Answer from the drawing. Dimensions are ordinates in mm from the lowest x, y and z of the part. A direction names the side the tool comes from. Coordinates: 2 decimals unless noted, no trailing zeros. Order: outer loops, then holes, each group sorted by start corner. A loop starts at its lowest first (then second) coordinate and runs counter-clockwise, first axis right, second up. Notation, with made-up numbers: M 81,-38 L 92,-38 A15 ccw 92,-22 Z; hole C -14.5,38.5 d1. An arc over 180 degrees is marked long. Write each question's results on one line, items separated by ' | '.
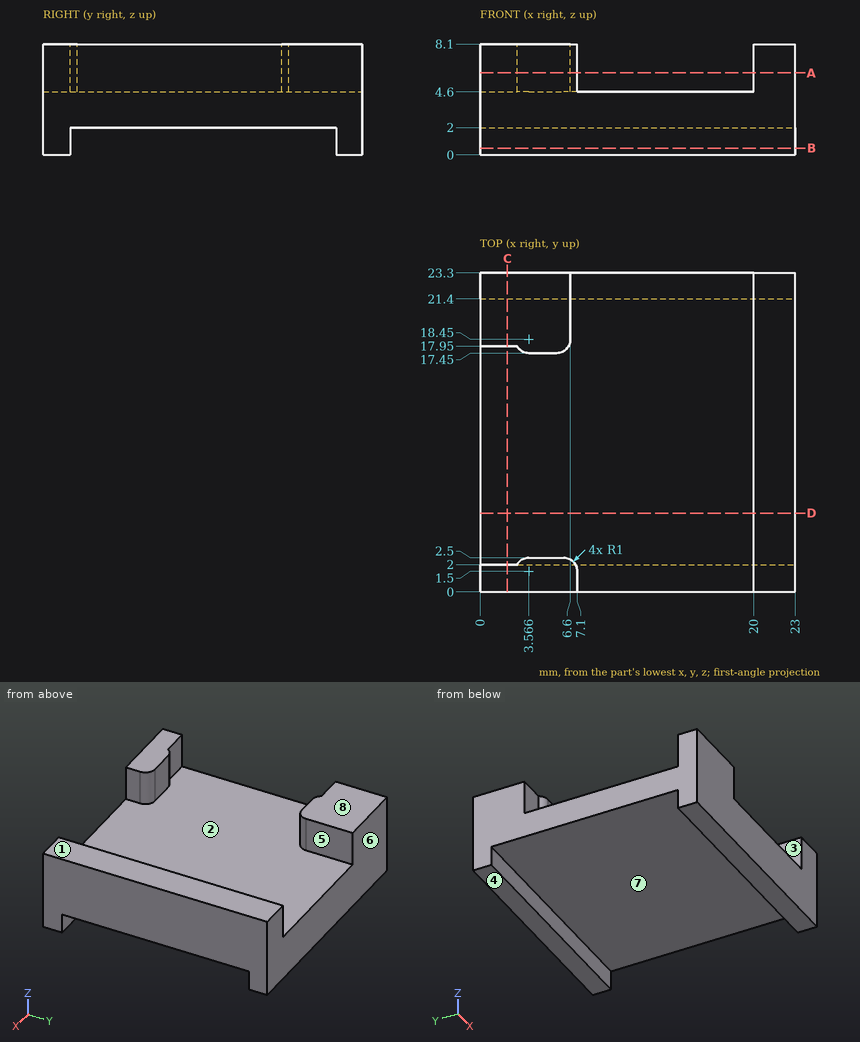
(1) The part is cut by section D-D, the plane y = 5.75. Write down the section's boundary in (x, z).
Conclusion:
outline: M 0,2 L 23,2 L 23,8.1 L 20,8.1 L 20,4.6 L 0,4.6 Z
(2) The part is cut by section A-A, the plane z = 6. Write down the section's boundary in (x, y), then the cut area to 3 significant figures.
Conclusion:
outline: M 0,0 L 7.1,0 L 7.1,1.5 A1 ccw 6.1,2.5 L 3.57,2.5 A1 ccw 2.7,2 L 0,2 Z; M 0,17.95 L 2.7,17.95 A1 ccw 3.57,17.45 L 5.6,17.45 A1 ccw 6.6,18.45 L 6.6,23.3 L 0,23.3 Z; M 20,0 L 23,0 L 23,23.3 L 20,23.3 Z | area: 123 mm²
(3) The part is cut by section B-B, the plane z = 0.5. Write down the section's boundary in (x, y), then the cut area to 3 significant figures.
Conclusion:
outline: M 0,0 L 23,0 L 23,2 L 0,2 Z; M 0,21.4 L 23,21.4 L 23,23.3 L 0,23.3 Z | area: 89.7 mm²
(4) Straight lines are drawn through the part: line 1 (Y direction, x = 3.5, z = 6); line 2 (Y direction, x = 15, z = 1.75); line 3 (Z direction, x = 13.75, y = 21.5). For each, find the intervals that lie inside material, in ascending order.
Conclusion:
line 1: 0 to 2.5, 17.45 to 23.3 | line 2: 0 to 2, 21.4 to 23.3 | line 3: 0 to 4.6
(5) The part is cut by section C-C, the plane x = 2. Write down the section's boundary in (y, z), then the cut area to 3 significant figures.
Conclusion:
outline: M 0,0 L 2,0 L 2,2 L 21.4,2 L 21.4,0 L 23.3,0 L 23.3,8.1 L 17.95,8.1 L 17.95,4.6 L 2,4.6 L 2,8.1 L 0,8.1 Z | area: 94.1 mm²
(6) For the marked faces 1, 2, 3, 4 and 5, determine the directions among +Z, -Z, +X, -X, +Y, -Y from which every point of the face is accessible in a straight line to the end or side of a thin tool.
Conclusion:
face 1: +Z, +X, -X, +Y, -Y | face 2: +Z | face 3: +Z, +Y, -Y | face 4: -Z, +X, -X, +Y, -Y | face 5: +Z, +Y
(7) The mould has two halves that part along Y. Classify the marked faces 6, 7 and 8: pulls with the +Y half, pulls with the -Y half, needs draft (parallel to the pull), parting line crosses it, or undercut.
Conclusion:
face 6: pulls with the +Y half | face 7: undercut | face 8: needs draft
(8) Given pin 1 (1 mm diameter, centred on x = 5, z = 6.5, fed in from -Y); pin 2 (5 mm diameter, centred on x = 18.5, y = 17, fed in from -Z); pin 3 (3 mm diameter, centred on x = 11, y = 6, fed in from +Z), each flat-ended and moving along its own axis, determine where each tip first touches the part or whether it passes through.
Conclusion:
pin 1: y = 0 | pin 2: z = 2 | pin 3: z = 4.6
